The model under review builds one solid part; all positions refer to its coordinate system, in mm. Face numbers are marked on the shaded views. A direction names the side the tool comes from. Round coordinates to 2 decimals unless told otherwise and drop trailing zeros. Write each loop counter-clockwise with the first axis right and the second up, starting at its lowest first coordinate (ties: lowest second). Pieces come first, ordered by that corner, then holes. Notation, with made-up numbers: (-30.5, 72.25) -> (24.5, 72.25) arc R30 cw to (24.5, 109.25) -> close; hole circle Ø7 at (31, -35). An arc over 180 degrees is marked (long way). Return JSON: item names as keys, results as strings. Group by question number.
1. Clearance check with flat-ended pins moving along their axes: P1, Ø1.4, axis at x = 0, y = -5, coming from the +Z side; P2, Ø1.5, axis at y = 8, z = 0.5, coming from the +X side; P3, Ø0.6, axis at x = 5, z = -1, coming from the -Y side. State where each tip first meets the part, or that it passes through.
2. Tool access review of the marked faces 4, 5, 6 and 7: name each direction out of +Z, -Z, +X, -X, +Y, -Y from which nothing blocks a thin tool from reaching the whole face with its end or side.
3. Take a section at B-B, the plane z = -0.9. Give the number of separate pieces and of enclosed holes in the cut face, then the cut area to 3 significant figures.
4. Mouldability with a two-part tool opening along X and no side actions: class the marked faces 1, 2 and 3 as pulls with the +X half, pulls with the -X half, needs draft (parallel to the pull), parting line crosses it, or undercut.
5. Take a section at D-D, the plane z = 0.8. Write out the cut boundary in (x, y).
6. For line 1 along X through (y, z) = (13.5, -1.55) (3 decimals); line 2 along Z through (x, y) = (-1.5, 5); line 3 along X through (y, z) = (8.5, -0.95) (3 decimals), list the stretches that pass through material, from the lowest coordinate up. Write a range as from..to.
7. Take a section at C-C, the plane x = 2.75. Write out the cut boundary in (y, z).
8. Take a section at A-A, the plane y = -7. Write out the cut boundary in (x, z) (3 decimals), then the cut area to 3 significant figures.
Autodesk Fusion 360 part; units mm, degrees
sketch "Sketch1" plane through (0, 0, 0) normal (0, 0, 1) x (1, 0, 0)
  circle A0 centre (0, 0) radius 3.5
  circle A1 centre (0, 0) radius 2.25
  circle A2 centre (0, 16.5) radius 2
  circle A3 centre (0, -14.5) radius 2
  circle A4 centre (-6.375, 0) radius 2
  circle A5 centre (6.375, 0) radius 2
  line L0 (0, 0) -> (0, 16.5) construction
  line L1 (-1.9917, 16.6818) -> (-3.4855, 0.3182)
  line L2 (-1.9893, -14.7069) -> (-3.4812, -0.3621)
  line L3 (1.9917, 16.6818) -> (3.4855, 0.3182)
  line L4 (1.9893, -14.7069) -> (3.4812, -0.3621)
  line L5 (-6.375, 2) -> (6.375, 2)
  line L6 (6.375, 2) -> (6.375, -2) construction
  line L7 (6.375, -2) -> (-6.375, -2)
  line L8 (-6.375, -2) -> (-6.375, 2) construction
  circle A6 centre (0, 0) radius 1.25
  circle A7 centre (0, 5) radius 0.625
  circle A8 centre (0, 7) radius 0.625
  circle A9 centre (0, 9) radius 0.625
  circle A10 centre (0, 11) radius 0.625
  circle A11 centre (0, 13) radius 0.625
  circle A12 centre (0, 15) radius 0.625
  circle A13 centre (0, 17) radius 0.625
  circle A14 centre (0, -5) radius 0.625
  circle A15 centre (0, -7) radius 0.625
  circle A16 centre (0, -9) radius 0.625
  circle A17 centre (0, -11) radius 0.625
  circle A18 centre (0, -13) radius 0.625
  circle A19 centre (0, -15) radius 0.625
  point P0 (0, -16.5)
  point P1 (0, 18.5)
  point P2 (-8.375, 0)
  point P3 (8.375, 0)
  dimension "d1" = 7
  dimension "d2" = 4.5
  dimension "d5" = 35
  dimension "d7" = 4
  dimension "d8" = 16.75
  dimension "d9" = 14.5
  dimension "d12" = 2.5
  dimension "d14" = 5
  dimension "d15" = 1.25
  dimension "d16" = 2
  dimension "d17" = 2
  dimension "d18" = 2
  dimension "d19" = 2
  dimension "d20" = 2
  dimension "d21" = 2
  dimension "d22" = 5
  dimension "d23" = 2
  dimension "d24" = 2
  dimension "d25" = 2
  dimension "d26" = 2
  dimension "d27" = 2
extrude "Extrude1" add sketch "Sketch1" along normal blind 2.5 contours A0 A1 L5 L7 | A0 A1 L5 | A0 A1 L7 | A0 A1 L5 L7
extrude "Extrude2" add sketch "Sketch1" against normal blind 2 contours A0 A1 L5 L7 | A0 A5 L3 L4 L5 L7 | A0 L3 L5 | A0 L4 L7 | A0 A1 L5 | A0 A2 L1 L3 L5 A12 | A0 A3 L2 L4 L7 A18 | A0 A1 L7 | A0 A1 L5 L7 | A0 L1 L5 | A1 L5 | A1 L5 L7 | A2 A12 | A5 | A0 L2 L7 | A1 L7 | A3 A18 | A0 A4 L1 L2 L5 L7 | A4 | A2 A12 | A2 A12 | A3 A18 | A3 A18 | A6 | A7 | A8 | A9 | A10 | A11 | A13 | A14 | A15 | A16 | A17 | A19
extrude "Extrude3" cut sketch "Sketch1" against normal through all contours A2 A12 | A2 A12 | A3 A18 | A3 A18 | A6 | A7 | A8 | A9 | A10 | A11 | A13 | A14 | A15 | A16 | A17 | A19 picked at (-0.0144, 14.4623) picked at (-0.0082, 14.8783) picked at (0.0144, -12.4623) picked at (-0.0082, -12.8783)
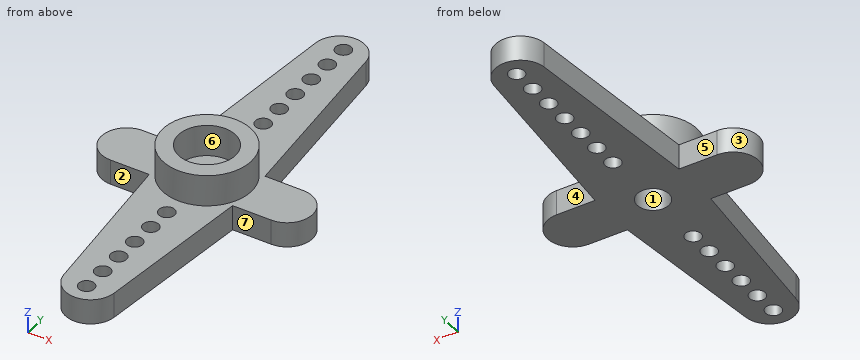
Output:
{
 "1": {"P1": "stops at z = 0", "P2": "stops at x = 2.84", "P3": "stops at y = -2"},
 "2": {"face 4": "+Z, -Z, +X, +Y", "face 5": "+Z, -Z, -X, +Y", "face 6": "+Z", "face 7": "+Z, -Z, +X, -Y"},
 "3": {"separate pieces": "1", "enclosed holes": "14", "area": "199 mm^2"},
 "4": {"face 1": "undercut", "face 2": "needs draft", "face 3": "pulls with the -X half"},
 "5": {"outline": "circle Ø7 at (0, 0); hole circle Ø4.5 at (0, 0)"},
 "6": {"line 1": "x = -2.282..-0.375, 0.375..2.282", "line 2": "z = -2..0", "line 3": "x = -2.739..-0.375, 0.375..2.739"},
 "7": {"outline": "(-7.39, -2) -> (8.38, -2) -> (8.38, 0) -> (2.17, 0) -> (2.17, 2.5) -> (-2.17, 2.5) -> (-2.17, 0) -> (-7.39, 0) -> close"},
 "8": {"outline": "(-2.791, -2) -> (-0.625, -2) -> (-0.625, 0) -> (-2.791, 0) -> close; (0.625, -2) -> (2.791, -2) -> (2.791, 0) -> (0.625, 0) -> close", "area": "8.66 mm^2"}
}
